Geometry check sheet. Reference: drawing and pictorial views, mm from the part's lowest x, y, z. Give positions to 0.01 mm unless a question says otherwise; leave off trailing zeros. Order: outer loops, then holes, each group sorted by start corner. A loop starts at its lowest first (then second) coordinate and runs counter-clockwise, first axis right, second up.
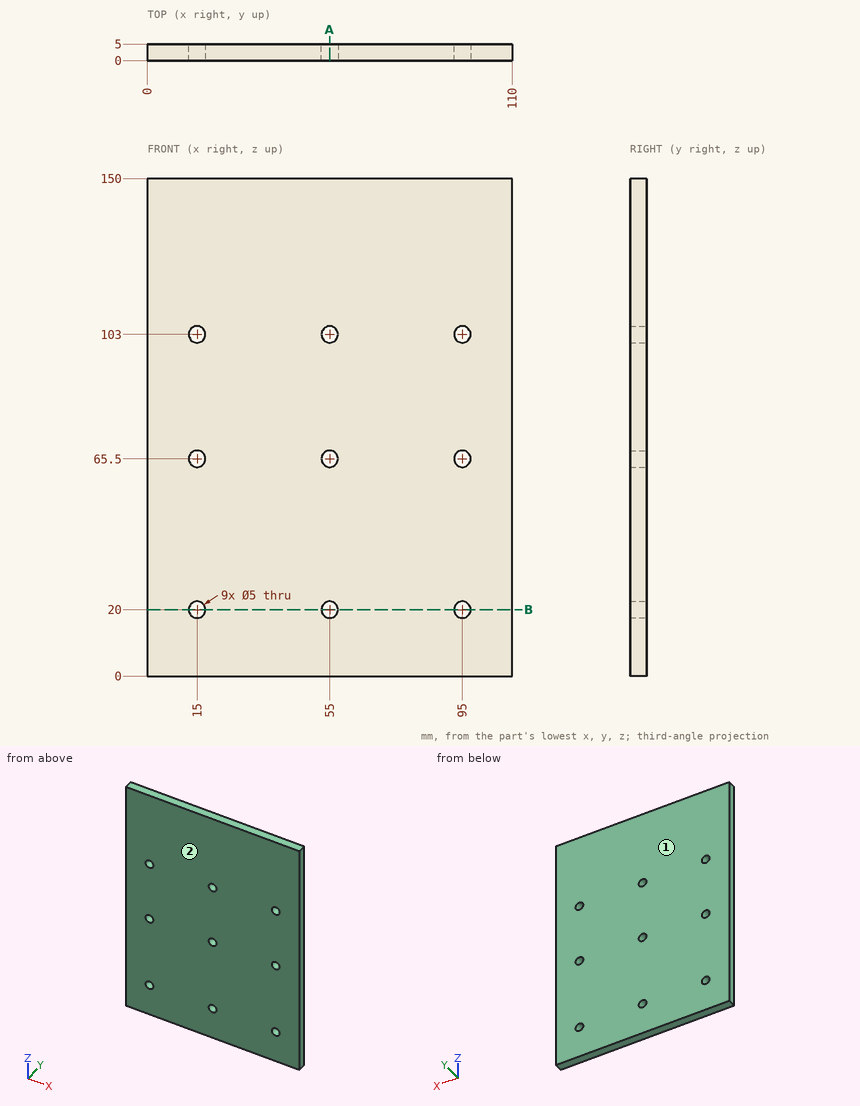
(1) Cross-section at A-A on x = 55. Enter the section's corners in (y, z).
Response values:
outline: (0, 0) - (5, 0) - (5, 17.5) - (0, 17.5) - close; (0, 22.5) - (5, 22.5) - (5, 63) - (0, 63) - close; (0, 68) - (5, 68) - (5, 100.5) - (0, 100.5) - close; (0, 105.5) - (5, 105.5) - (5, 150) - (0, 150) - close
(2) Gauge pin test, flat end, axial feed: pin 1 Ø3 at (x, z) = (55, 20) entering from +Y. Record the tip position at first contact, or that the pin passes through.
Response values:
pin 1: passes through
(3) Cross-section at B-B on z = 20. Enter the section's corners in (x, y), then the cut area to 3 significant figures.
Response values:
outline: (0, 0) - (12.5, 0) - (12.5, 5) - (0, 5) - close; (17.5, 0) - (52.5, 0) - (52.5, 5) - (17.5, 5) - close; (57.5, 0) - (92.5, 0) - (92.5, 5) - (57.5, 5) - close; (97.5, 0) - (110, 0) - (110, 5) - (97.5, 5) - close
area: 475 mm2
(4) Material ranges on L1, parallel to Z at x = 55, y = 2.8; L2, parallel to X at y = 0.4, z = 63.5, recorded low to high.
Response values:
L1: z = 0 to 17.5, 22.5 to 63, 68 to 100.5, 105.5 to 150
L2: x = 0 to 13.5, 16.5 to 53.5, 56.5 to 93.5, 96.5 to 110
(5) Release check for a two-part mould opening along Y. For the marked faces 1 and 2 record: released by +Y, released by -Y, zero draft, split by the parting line, or undercut.
Response values:
face 1: released by +Y
face 2: released by -Y
